Build history of the part. All positions in model axes, mm. Face numbers are marked on the shaded views. Round coordinates to 2 decimals unless told otherwise and drop trailing zeros. Write each loop counter-clockwise with the first axis right and the second up, starting at its lowest first coordinate (ties: lowest second). Pieces come first, ordered by that corner, then holes. Notation, with made-up numbers: (13.5, 52.25) -> (58.5, 52.25) arc R21 cw to (58.5, 65.25) -> close; hole circle Ø9 at (68.25, -11). An arc over 180 degrees is marked (long way). Answer in a Markdown table with one row per item.
```python
from build123d import *

# Parameters (mm, degrees)
SKETCH1_W           = 110
SKETCH1_H           = 110
BOSS_EXTRUDE1_DEPTH = 3
FILLET1_R           = 5
SKETCH2_R           = 5
BOSS_EXTRUDE2_DEPTH = 3
SKETCH6_R           = 1.55
CUT_EXTRUDE1_DEPTH  = 7


with BuildPart() as part:
    # Sketch1 → Boss-Extrude1 (new body)
    with BuildSketch(Plane(origin=(0, 0, 0), x_dir=(1, 0, 0), z_dir=(0, 1, 0))):
        Rectangle(SKETCH1_W, SKETCH1_H)
    extrude(amount=BOSS_EXTRUDE1_DEPTH)

    # Fillet1
    fillet1_edges = [part.edges().sort_by_distance(p)[0] for p in [
        (-55, 1.5, -55),
        (55, 1.5, -55),
        (55, 1.5, 55),
        (-55, 1.5, 55),
    ]]
    fillet(fillet1_edges, radius=FILLET1_R)

    # Sketch2 → Boss-Extrude2 (add)
    with BuildSketch(Plane(origin=(0, 3, 0), x_dir=(1, 0, 0), z_dir=(0, 1, 0))):
        with Locations((-50, 50)):
            Circle(SKETCH2_R)
        with Locations((50, 50)):
            Circle(SKETCH2_R)
        with Locations((50, -50)):
            Circle(SKETCH2_R)
        with Locations((-50, -50)):
            Circle(SKETCH2_R)
    extrude(amount=BOSS_EXTRUDE2_DEPTH)

    # Sketch6 → Cut-Extrude1 (cut, through all)
    with BuildSketch(Plane.XZ):
        with Locations((-50, 50)):
            Circle(SKETCH6_R)
        with Locations((50, -50)):
            Circle(SKETCH6_R)
        with Locations((50, 50)):
            Circle(SKETCH6_R)
        with Locations((-50, -50)):
            Circle(SKETCH6_R)
    extrude(amount=-CUT_EXTRUDE1_DEPTH, mode=Mode.SUBTRACT)


solid = part.part
```
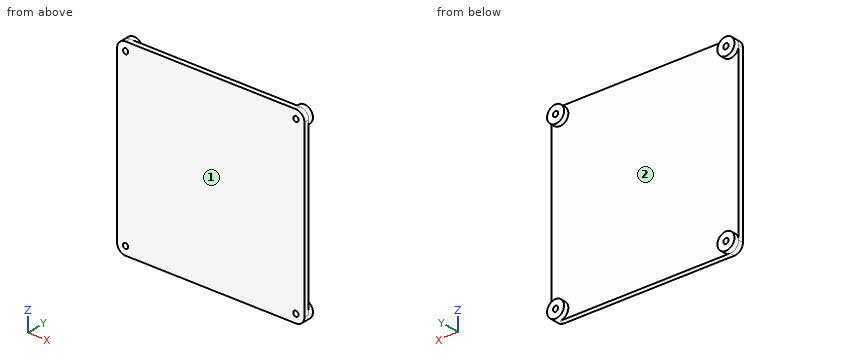
Q1. Drop flat-ended pins along their axis: P1, Ø10, axis at x = 20.5, z = -4, coming from the -Y side; P2, Ø8, axis at x = -9, z = 11.5, coming from the +Y side. Give the stop position or say it passes through.
A:
| item | result |
|---|---|
| P1 | y = 0 |
| P2 | y = 3 |
Q2. Saw through at B-B on z = -11. Write the cut outline in (x, y), plus the area to 3 significant figures.
A:
| item | result |
|---|---|
| outline | (-55, 0) -> (55, 0) -> (55, 3) -> (-55, 3) -> close |
| area | 330 mm² |
Q3. Two-plate mould, pull along Z, no slides. Class the marked faces 1 and 2: released by +Z, released by -Z, zero draft, split by the parting line, or undercut.
A:
| item | result |
|---|---|
| face 1 | zero draft |
| face 2 | undercut |
Q4. Wall check: line 1 (Z direction, x = 50, y = 4.45); line 2 (Y direction, x = 40.5, z = 25.5); line 3 (X direction, y = 4.55, z = -48). Give the ranges that are in metal, low to high. Write a range as [from, to].
A:
| item | result |
|---|---|
| line 1 | [-55, -51.55], [-48.45, -45], [45, 48.45], [51.55, 55] |
| line 2 | [0, 3] |
| line 3 | [-54.58, -45.42], [45.42, 54.58] |
Q5. Saw through at A-A on x = 32. Write the cut outline in (y, z), plus the area to 3 significant figures.
A:
| item | result |
|---|---|
| outline | (0, -55) -> (3, -55) -> (3, 55) -> (0, 55) -> close |
| area | 330 mm² |
